Verification items for the finished model (mm, model axes). Give positions to 0.01 mm unless a question says otherwise; leave off trailing zeros. Write each loop counter-clockwise with the first axis right and the second up, starting at its lowest first coordinate (ties: lowest second). Pieces come first, ordered by that corner, then holes. Notation, with made-up numbers: (84, 79) -> (124, 79) arc R23 cw to (124, 105) -> close; hole circle Ø7 at (2.25, 18). An arc over 180 degrees is marked (long way). Answer as CSV lines item,"result". Start each with the question number.
1) Material ranges on L1, parallel to Z at x = 3, y = -18.5; L2, parallel to X at y = 2, z = -530; L3, parallel to Y at x = -2.5, z = 484, recorded low to high.
2) Sectioned sample at C-C on z = 109.5. Record the cut outline in (x, y).
3) Sectioned sample at A-A on y = 0. Record the cut outline in (x, z).
4) Gauge pin test, flat ends, axial feed: pin 1 Ø6 at (x, y) = (-15, -14) entering from -Z; pin 2 Ø2 at (y, z) = (32.5, 336) entering from +X; pin 3 Ø5 at (y, z) = (11, 10) entering from -X. Record the tip position at first contact, or that the pin passes through.
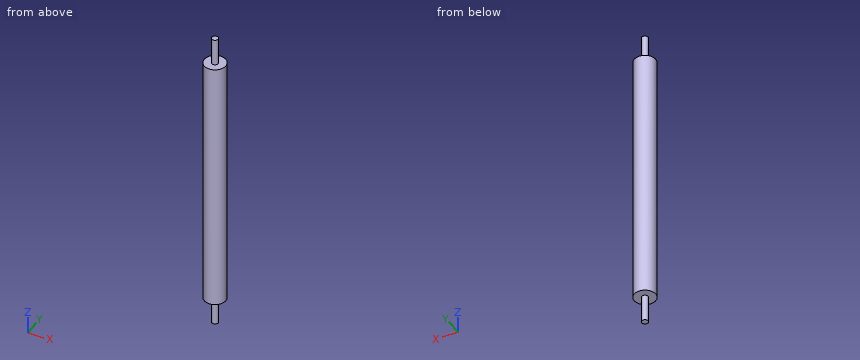
```python
from build123d import *

# Parameters (mm, degrees)
SKETCH1_R           = 50
BOSS_EXTRUDE1_DEPTH = 600
BOSS_EXTRUDE2_DEPTH = 600
BOSS_EXTRUDE4_START = 600
SKETCH6_R           = 15
BOSS_EXTRUDE4_DEPTH = 125


with BuildPart() as part:
    # Sketch1 → Boss-Extrude1 (new, symmetric)
    with BuildSketch(Plane.XY):
        Circle(SKETCH1_R)
    extrude(amount=BOSS_EXTRUDE1_DEPTH, both=True)

    # Sketch4 → Boss-Extrude2 (add, symmetric)
    with BuildSketch(Plane.XY):
        with BuildLine():
            Line((-5, 14.142135624), (-5, 18.3))
            Line((-5, 18.3), (5, 18.3))
            Line((5, 18.3), (5, 14.142135624))
            ThreePointArc((5, 14.142135624), (0, -15), (-5, 14.142135624))
        make_face()
    extrude(amount=BOSS_EXTRUDE2_DEPTH, both=True)

    # Sketch6 → Boss-Extrude4 (add)
    with BuildSketch(Plane.XY.offset(BOSS_EXTRUDE4_START)):
        Circle(SKETCH6_R)
    boss_extrude4 = extrude(amount=BOSS_EXTRUDE4_DEPTH)

    # Mirror1: Boss-Extrude4 across plane
    add(boss_extrude4.mirror(Plane.XY))


solid = part.part
```
Ans:
1,L1,"z = -600 to 600"
1,L2,"x = -49.96 to 49.96"
1,L3,"y = -49.94 to 49.94"
2,outline,"circle Ø100 at (0, 0)"
3,outline,"(-50, -600) -> (-15, -600) -> (-15, -725) -> (15, -725) -> (15, -600) -> (50, -600) -> (50, 600) -> (15, 600) -> (15, 725) -> (-15, 725) -> (-15, 600) -> (-50, 600) -> close"
4,pin 1,"stops at z = -600"
4,pin 2,"stops at x = 38.83"
4,pin 3,"stops at x = -49.27"
